Input: part model. Units: mm. Frame: model coordinates. A direction names the side the tool comes from. Give positions to 0.01 mm unless a question says otherwise; leave off trailing zeros. Order: outer loops, then holes, each group sorted by start corner. A loop starts at its lowest first (then second) coordinate and runs counter-clockwise, first axis right, second up. Notation, with made-up numbers: (-31.75, 69.5) - (12.25, 69.5) arc R9 ccw to (12.25, 77.5) - close; hole circle Ø11 at (47, 2.5). An arc over 180 degrees is marked (long way). Use a Markdown table: item, result.
Autodesk Inventor part; units mm, degrees
ref_plane "YZ Plane" through (0, 0, 0) normal (1, 0, 0) x (0, 1, 0)
ref_plane "XZ Plane" through (0, 0, 0) normal (0, 1, 0) x (-1, 0, 0)
ref_plane "XY Plane" through (0, 0, 0) normal (0, 0, 1) x (1, 0, 0)
sketch "Sketch1" plane through (0, 0, 0) normal (1, 0, 0) x (0, 1, 0)
  line L0 (-7.458, 13.2905) -> (-7.458, -13.2905)
  arc A0 (-7.458, -9.5323) -> (-7.458, 9.5323) centre (0, 0) ccw
  arc A1 (-7.458, -13.2905) -> (-7.458, 13.2905) centre (0, 0) ccw
  point P0 (0, 0)
extrude "Extrusion1" add sketch "Sketch1" along normal blind 9.906 contours A1 L0 A0
sketch "Sketch2" plane through (0, -7.458, 9.5323) normal (0, -1, 0) x (1, 0, 0)
  line L0 (9.906, 3.7582) -> (9.906, 0)
  line L1 (9.906, 3.7582) -> (0, 3.7582)
  line L2 (0, 3.7582) -> (0, 0)
  line L3 (0, 0) -> (9.906, 0)
  line L4 (9.906, 0) -> (9.906, 3.7582)
  point P0 (0, -9.5323)
extrude "Extrusion2" add sketch "Sketch2" along normal blind 22.9108
sketch "Sketch3" plane through (0, -7.458, -13.2905) normal (0, -1, 0) x (1, 0, 0)
  line L0 (9.906, 3.7582) -> (9.906, 0)
  line L1 (9.906, 3.7582) -> (0, 3.7582)
  line L2 (0, 3.7582) -> (0, 0)
  line L3 (0, 0) -> (9.906, 0)
  line L4 (9.906, 0) -> (9.906, 3.7582)
  point P0 (0, 13.2905)
extrude "Extrusion3" add sketch "Sketch3" along normal blind 22.9108
fillet "Fillet1" radius 10.16 1 edges at (4.953, -7.458, -9.5323)
fillet "Fillet2" radius 10.16 1 edges at (4.953, -7.458, 9.5323)
fillet "Fillet3" radius 10.16 1 edges at (4.953, -7.458, 13.2905)
fillet "Fillet4" radius 10.16 1 edges at (4.953, -7.458, -13.2905)
sketch "Sketch5" plane through (9.906, 0, 0) normal (1, 0, 0) x (0, 0, -1)
  point P0 (0, 0)
properties part number "eye motor holder2_3DPrint"
1. Section query D-D (z = 0). Return loops of the section in (x, y), then the cut area to 3 significant figures.
Response:
| item | result |
|---|---|
| outline | (0, 12.1) - (9.91, 12.1) - (9.91, 15.24) - (0, 15.24) - close |
| area | 31.1 mm^2 |
2. Pin query (flat end, axial travel): pin 1 (3 mm diameter, centred on x = 3.5, y = -21.5, fed in from +Z); pin 2 (3 mm diameter, centred on x = 6.5, z = 6.5, fed in from -Y); pin 3 (5 mm diameter, centred on x = 7.5, y = -23.5, fed in from -Z). Return the tip coordinate at first contact, or that it passes through.
Response:
| item | result |
|---|---|
| pin 1 | stops at z = 13.29 |
| pin 2 | stops at y = 9.08 |
| pin 3 | stops at z = -13.29 |
3. Set-up query: faces 4 (the face through (5, -20, -9.532)), 5 (the face through (0, -9, 10)), 6 (the face through (5, -20, -13.29)), 7 (the face through (5.02, -7.98, 9.82)). Return all of +Z, -Z, +X, -X, +Y, -Y with unobstructed straight access to the full face (end or side cutting, diameter ignored); none if empty.
Response:
| item | result |
|---|---|
| face 4 | +X, -X, -Y |
| face 5 | +Z, -Z, -X, +Y, -Y |
| face 6 | -Z, +X, -X, -Y |
| face 7 | +X, -X |
4. Section query B-B (x = 2.25). Return loops of the section in (y, z).
Response:
| item | result |
|---|---|
| outline | (-30.37, -13.29) - (-9.76, -13.29) arc R10.16 cw to (-5.86, -14.07) arc R15.24 ccw (long way) to (-5.86, 14.07) arc R10.16 cw to (-9.76, 13.29) - (-30.37, 13.29) - (-30.37, 9.53) - (-10.39, 9.53) arc R10.16 ccw to (-5.65, 10.71) arc R12.1 cw (long way) to (-5.65, -10.71) arc R10.16 ccw to (-10.39, -9.53) - (-30.37, -9.53) - close |
5. Section query A-A (y = 0). Return loops of the section in (x, z), then the cut area to 3 significant figures.
Response:
| item | result |
|---|---|
| outline | (0, -15.24) - (9.91, -15.24) - (9.91, -12.1) - (0, -12.1) - close; (0, 12.1) - (9.91, 12.1) - (9.91, 15.24) - (0, 15.24) - close |
| area | 62.1 mm^2 |
6. Section query C-C (y = -25.5). Return loops of the section in (x, z).
Response:
| item | result |
|---|---|
| outline | (0, -13.29) - (9.91, -13.29) - (9.91, -9.53) - (0, -9.53) - close; (0, 9.53) - (9.91, 9.53) - (9.91, 13.29) - (0, 13.29) - close |
7. Mould query, pull axis Z, two halves, no side actions, for faces 1 (the face through (5, -20, 13.29)), 2 (the face through (9.906, -9, 10)), 3 (the face through (4.9, 12.1, 0.3)). Classes: pulls with the +Z half, pulls with the -Z half, needs draft (parallel to the pull), parting line crosses it, or undercut.
Response:
| item | result |
|---|---|
| face 1 | pulls with the +Z half |
| face 2 | needs draft |
| face 3 | undercut |
8. Material intervals for line 1 along Z through (x, y) = (2.5, -17); line 2 along Z through (x, y) = (6, 0); line 3 along Y through (x, z) = (3, -11), sorted ascending.
Response:
| item | result |
|---|---|
| line 1 | z = -13.29 to -9.53, 9.53 to 13.29 |
| line 2 | z = -15.24 to -12.1, 12.1 to 15.24 |
| line 3 | y = -30.37 to -5.05, 5.05 to 10.55 |
